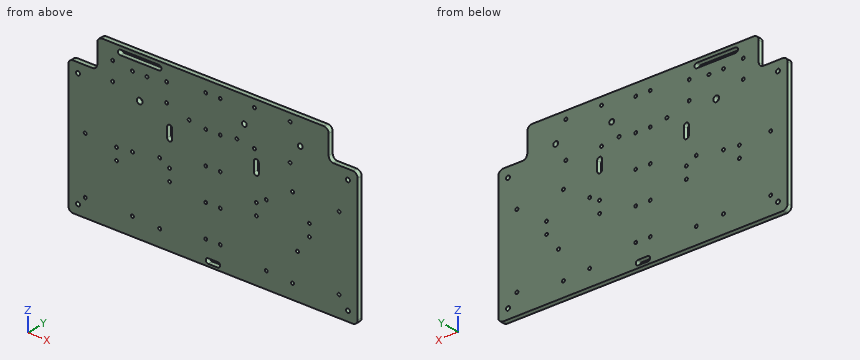
```python
from build123d import *

# Parameters (mm, degrees)
ESQUISSE1_R             = 2.05
ESQUISSE1_R_2           = 1.55
ESQUISSE1_R_3           = 2.5
ESQUISSE1_R_4           = 3
BOSS_EXTRU_1_DEPTH      = 5
CONG_2_R                = 5
ESQUISSE2_R             = 1.5
ENL_V_MAT_EXTRU_1_DEPTH = 10


with BuildPart() as part:
    # Esquisse1 → Boss.-Extru.1 (new body)
    with BuildSketch(Plane(origin=(0, 0, 0), x_dir=(1, 0, 0), z_dir=(0, 1, 0))):
        Polygon((150, -69), (150, 69), (-149.848840409, 69), (-150, 69), (-150, -69), (-120, -69), (-120, -99), (120, -99), (120, -69), align=None)
        with Locations(Location((-140, 59, 0), (0, 0, 270))):
            Circle(ESQUISSE1_R, mode=Mode.SUBTRACT)
        with Locations(Location((140, 59, 0), (0, 0, 90))):
            Circle(ESQUISSE1_R, mode=Mode.SUBTRACT)
        with Locations(Location((140, -59, 0), (0, 0, 270))):
            Circle(ESQUISSE1_R, mode=Mode.SUBTRACT)
        with Locations(Location((-140, -59, 0), (0, 0, 90))):
            Circle(ESQUISSE1_R, mode=Mode.SUBTRACT)
        with Locations(Location((-48, -83, 0), (0, 0, 270))):
            Circle(ESQUISSE1_R_2, mode=Mode.SUBTRACT)
        with Locations(Location((-104, -83, 0), (0, 0, 270))):
            Circle(ESQUISSE1_R_2, mode=Mode.SUBTRACT)
        with Locations(Location((-48, -64, 0), (0, 0, 270))):
            Circle(ESQUISSE1_R_2, mode=Mode.SUBTRACT)
        with Locations(Location((-104, -64, 0), (0, 0, 270))):
            Circle(ESQUISSE1_R_2, mode=Mode.SUBTRACT)
        with Locations(Location((82.54, -28.63, 0), (0, 0, 270))):
            Circle(ESQUISSE1_R_2, mode=Mode.SUBTRACT)
        with Locations(Location((130.8, -27.36, 0), (0, 0, 270))):
            Circle(ESQUISSE1_R_2, mode=Mode.SUBTRACT)
        with Locations(Location((130.8, 47.57, 0), (0, 0, 270))):
            Circle(ESQUISSE1_R_2, mode=Mode.SUBTRACT)
        with Locations(Location((82.54, 53.92, 0), (0, 0, 270))):
            Circle(ESQUISSE1_R_2, mode=Mode.SUBTRACT)
        with Locations(Location((87.62, 23.44, 0), (0, 0, 270))):
            Circle(ESQUISSE1_R_2, mode=Mode.SUBTRACT)
        with Locations(Location((43, -54, 0), (0, 0, 270))):
            Circle(ESQUISSE1_R_2, mode=Mode.SUBTRACT)
        with Locations(Location((80, -54, 0), (0, 0, 270))):
            Circle(ESQUISSE1_R_2, mode=Mode.SUBTRACT)
        with Locations(Location((80, -91, 0), (0, 0, 270))):
            Circle(ESQUISSE1_R_2, mode=Mode.SUBTRACT)
        with Locations(Location((43, -91, 0), (0, 0, 270))):
            Circle(ESQUISSE1_R_2, mode=Mode.SUBTRACT)
        with Locations(Location((-132.5, 50.5, 0), (0, 0, 270))):
            Circle(ESQUISSE1_R_2, mode=Mode.SUBTRACT)
        with Locations(Location((-132.5, -7.5, 0), (0, 0, 270))):
            Circle(ESQUISSE1_R_2, mode=Mode.SUBTRACT)
        with Locations(Location((-83.5, -7.5, 0), (0, 0, 270))):
            Circle(ESQUISSE1_R_2, mode=Mode.SUBTRACT)
        with Locations(Location((-83.5, 50.5, 0), (0, 0, 270))):
            Circle(ESQUISSE1_R_2, mode=Mode.SUBTRACT)
        with Locations(Location((-55.25, 52, 0), (0, 0, 270))):
            Circle(ESQUISSE1_R_2, mode=Mode.SUBTRACT)
        with Locations(Location((-55.25, -12, 0), (0, 0, 270))):
            Circle(ESQUISSE1_R_2, mode=Mode.SUBTRACT)
        with Locations(Location((55.25, 52, 0), (0, 0, 270))):
            Circle(ESQUISSE1_R_2, mode=Mode.SUBTRACT)
        with Locations(Location((55.25, -12, 0), (0, 0, 270))):
            Circle(ESQUISSE1_R_2, mode=Mode.SUBTRACT)
        with Locations(Location((-24.75, -56.5, 0), (0, 0, 270))):
            Circle(ESQUISSE1_R_2, mode=Mode.SUBTRACT)
        with Locations(Location((24.75, -56.5, 0), (0, 0, 270))):
            Circle(ESQUISSE1_R_2, mode=Mode.SUBTRACT)
        with Locations(Location((32.5, -72.5, 0), (0, 0, 270))):
            Circle(ESQUISSE1_R_3, mode=Mode.SUBTRACT)
        with Locations(Location((90.5, -72.5, 0), (0, 0, 270))):
            Circle(ESQUISSE1_R_3, mode=Mode.SUBTRACT)
        with Locations(Location((-76, -56, 0), (0, 0, 270))):
            Circle(ESQUISSE1_R_4, mode=Mode.SUBTRACT)
        with BuildLine():
            Line((-56, -95.5), (-96, -95.5))
            ThreePointArc((-96, -95.5), (-98.5, -93), (-96, -90.5))
            Line((-96, -90.5), (-56, -90.5))
            ThreePointArc((-56, -90.5), (-53.5, -93), (-56, -95.5))
        make_face(mode=Mode.SUBTRACT)
        with BuildLine():
            Line((-5, 66.5), (5, 66.5))
            ThreePointArc((5, 66.5), (7.5, 64), (5, 61.5))
            Line((5, 61.5), (-5, 61.5))
            ThreePointArc((-5, 61.5), (-7.5, 64), (-5, 66.5))
        make_face(mode=Mode.SUBTRACT)
        with BuildLine():
            Line((-42.5, -32.709135822), (-42.5, -42.709135822))
            ThreePointArc((-42.5, -42.709135822), (-45, -45.209135822), (-47.5, -42.709135822))
            Line((-47.5, -42.709135822), (-47.5, -32.709135822))
            ThreePointArc((-47.5, -32.709135822), (-45, -30.209135822), (-42.5, -32.709135822))
        make_face(mode=Mode.SUBTRACT)
        with BuildLine():
            Line((42.5, -32.709135822), (42.5, -42.709135822))
            ThreePointArc((42.5, -42.709135822), (45, -45.209135822), (47.5, -42.709135822))
            Line((47.5, -42.709135822), (47.5, -32.709135822))
            ThreePointArc((47.5, -32.709135822), (45, -30.209135822), (42.5, -32.709135822))
        make_face(mode=Mode.SUBTRACT)
    extrude(amount=BOSS_EXTRU_1_DEPTH)

    # Congé2
    cong_2_edges = [part.edges().sort_by_distance(p)[0] for p in [
        (150, 2.5, -69),
        (150, 2.5, 69),
        (120, 2.5, 69),
        (120, 2.5, 99),
        (-120, 2.5, 99),
        (-120, 2.5, 69),
        (-150, 2.5, 69),
        (-150, 2.5, -69),
    ]]
    fillet(cong_2_edges, radius=CONG_2_R)

    # Esquisse2 → Enlèv. mat.-Extru.1 (cut)
    with BuildSketch(Plane(origin=(0, 5, 0), x_dir=(1, 0, 0), z_dir=(0, 1, 0))):
        with Locations(Location((-7.5, 45, 0), (0, 0, 270))):
            Circle(ESQUISSE2_R)
        with Locations(Location((7.5, 45, 0), (0, 0, 90))):
            Circle(ESQUISSE2_R)
        with Locations(Location((-7.5, 12, 0), (0, 0, 270))):
            Circle(ESQUISSE2_R)
        with Locations(Location((7.5, 12, 0), (0, 0, 90))):
            Circle(ESQUISSE2_R)
        with Locations(Location((-7.5, -21, 0), (0, 0, 270))):
            Circle(ESQUISSE2_R)
        with Locations(Location((7.5, -21, 0), (0, 0, 90))):
            Circle(ESQUISSE2_R)
        with Locations(Location((-7.5, -54, 0), (0, 0, 270))):
            Circle(ESQUISSE2_R)
        with Locations(Location((7.5, -54, 0), (0, 0, 90))):
            Circle(ESQUISSE2_R)
        with Locations(Location((-7.5, -87, 0), (0, 0, 270))):
            Circle(ESQUISSE2_R)
        with Locations(Location((7.5, -87, 0), (0, 0, 90))):
            Circle(ESQUISSE2_R)
        with Locations(Location((-100, 6, 0), (0, 0, 270))):
            Circle(ESQUISSE2_R)
        with Locations(Location((-100, -6, 0), (0, 0, 90))):
            Circle(ESQUISSE2_R)
        with Locations(Location((100, -6, 0), (0, 0, 270))):
            Circle(ESQUISSE2_R)
        with Locations(Location((100, 6, 0), (0, 0, 90))):
            Circle(ESQUISSE2_R)
        with Locations(Location((-83.5, -80.5, 0), (0, 0, 270))):
            Circle(ESQUISSE2_R)
        with Locations(Location((-68.5, -80.5, 0), (0, 0, 90))):
            Circle(ESQUISSE2_R)
        with Locations(Location((-45, -6, 0), (0, 0, 90))):
            Circle(ESQUISSE2_R)
        with Locations(Location((-45, 6, 0), (0, 0, 270))):
            Circle(ESQUISSE2_R)
        with Locations(Location((45, 6, 0), (0, 0, 90))):
            Circle(ESQUISSE2_R)
        with Locations(Location((45, -6, 0), (0, 0, 270))):
            Circle(ESQUISSE2_R)
    extrude(amount=-ENL_V_MAT_EXTRU_1_DEPTH, mode=Mode.SUBTRACT)


solid = part.part
```
Source: CAD feature listing. Evaluate the final solid. Frame: model axes, mm. Round coordinates to 2 decimals unless told otherwise and drop trailing zeros. Use a Markdown table: item, result. Add a question column.
1. Contact query for a flat-ended pin moving along its axis: P1, Ø3.5, axis at x = -140, z = 59, coming from the -Y side. Output: stop coordinate, or through.
2. Section query A-A on y = 1.05. Give the number of separate pieces and of enclosed holes in the cut face, then the cut area to 3 significant figures.
3. Line query: line 1 (X direction, y = 2.9, z = 37); line 2 (Z direction, x = 130.8, y = 3.65); line 3 (Z direction, x = -83.5, y = 1.25). Output: solid intervals per line, ascending.
Reported:
| question | item | result |
|---|---|---|
| 1 | P1 | passes through |
| 2 | separate pieces | 1 |
| 2 | enclosed holes | 54 |
| 2 | area | 47,700 mm² |
| 3 | line 1 | x = -150 to -47.5, -42.5 to 42.5, 47.5 to 150 |
| 3 | line 2 | z = -69 to -49.12, -46.02 to 25.81, 28.91 to 69 |
| 3 | line 3 | z = -69 to -52.05, -48.95 to 5.95, 9.05 to 79, 82 to 90.5, 95.5 to 99 |
